from build123d import *

# Parameters (mm, degrees)
SKETCH1_R           = 4.7625
SKETCH1_W           = 25
SKETCH1_H           = 10
BOSS_EXTRUDE1_DEPTH = 10
FILLET1_R           = 12


with BuildPart() as part:
    # Sketch1 → Boss-Extrude1 (new body)
    with BuildSketch(Plane.XY):
        Polygon((50, 0), (25, 35.703700169), (0, 0), align=None)
        with Locations((25, 15)):
            Circle(SKETCH1_R, mode=Mode.SUBTRACT)
        with Locations((25, -5)):
            Rectangle(SKETCH1_W, SKETCH1_H)
    extrude(amount=BOSS_EXTRUDE1_DEPTH)

    # Fillet1
    fillet1_edges = [part.edges().sort_by_distance(p)[0] for p in [
        (25, 35.703700169, 5),
    ]]
    fillet(fillet1_edges, radius=FILLET1_R)


solid = part.part
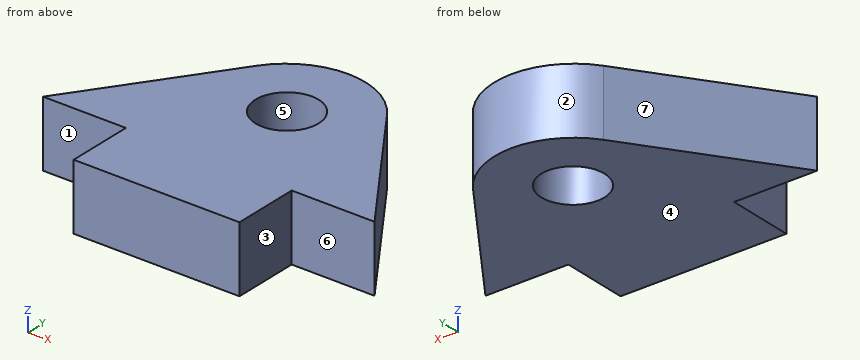
Read the model definition and answer for the solid it produces. Units are mm, in the model's axes. Face numbers are marked on the shaded views. A direction names the side the tool comes from. Round coordinates to 2 decimals unless told otherwise and drop trailing zeros. Write each loop counter-clockwise with the first axis right and the second up, starting at its lowest first coordinate (ties: lowest second). Pieces come first, ordered by that corner, then holes.
Q1. Flat-ended cylindrical pins translate along their axes: P1, Ø3, axis at y = -7, z = 6.5, coming from the +X side; P2, Ø5, axis at x = 4.5, z = 3, coming from the -Y side; P3, Ø3, axis at y = -4.5, z = 6, coming from the -X side; P4, Ø5.5, axis at x = 25, y = 15, coming from the -Z side. Find the tip coordinate at first contact, or state that the pin passes through.
Values:
P1: stops at x = 37.5
P2: stops at y = 0
P3: stops at x = 12.5
P4: passes through
Q2. The mould has two halves that part along Y. Classify the marked faces 4, 5, 6 and 7: released by +Y, released by -Y, zero draft, split by the parting line, or undercut.
Values:
face 4: zero draft
face 5: undercut
face 6: released by -Y
face 7: released by +Y
Q3. Find section A-A on z = 2. Determine the outline of the cut face in (x, y) (1 decimal).
Values:
outline: (0, 0) - (12.5, 0) - (12.5, -10) - (37.5, -10) - (37.5, 0) - (50, 0) - (34.8, 21.7) arc R12 ccw to (15.2, 21.7) - close; hole circle Ø9.5 at (25, 15)
Q4. Find section D-D on y = -2.5. Determine the outline of the cut face in (x, z).
Values:
outline: (12.5, 0) - (37.5, 0) - (37.5, 10) - (12.5, 10) - close
Q5. Straight lines are drawn through the part: line 1 (X direction, y = -5, z = 6.25); line 2 (X direction, y = 14.5, z = 3.5); line 3 (Y direction, x = 29, z = 6). For each, find the intervals that lie inside material, in ascending order.
Values:
line 1: x = 12.5 to 37.5
line 2: x = 10.15 to 20.26, 29.74 to 39.85
line 3: y = -10 to 12.42, 17.58 to 26.1
Q6. Find section C-C on x = 25. Determine the outline of the cut face in (y, z).
Values:
outline: (-10, 0) - (10.24, 0) - (10.24, 10) - (-10, 10) - close; (19.76, 0) - (26.78, 0) - (26.78, 10) - (19.76, 10) - close
Q7. A tool of negligible diameter and unlimited length cuts with its end or side. For the marked faces 1, 2 and 3, from which of +Z, -Z, +X, -X, +Y, -Y can it reach the whole face along a straight path? Write none if from no direction.
Values:
face 1: +Z, -Z, -X, -Y
face 2: +Z, -Z, +Y
face 3: +Z, -Z, +X, -Y
Q8. Find section B-B on y = 16. Determine the outline of the cut face in (x, z).
Values:
outline: (11.2, 0) - (20.34, 0) - (20.34, 10) - (11.2, 10) - close; (29.66, 0) - (38.8, 0) - (38.8, 10) - (29.66, 10) - close
